Job drawing, mm, ordinate dimensions from the low corner. One solid piece. A direction names the side the tool comes from. Give positions to 0.01 mm unless a question says otherwise; leave off trailing zeros. Order: outer loops, then holes, each group sorted by start corner. A loop starts at its lowest first (then second) coordinate and runs counter-clockwise, first axis right, second up. Notation, with made-up numbers: M 45,2.25 L 59,2.25 A23 ccw 59,23.25 Z; hole C 87,-36 d11. An arc over 180 degrees is marked long. Put each result on its own line as item: value. Start each with the question number.
1) Pin check, flat tip, straight feed: pin 1 (10 mm diameter, centred on y = 46.5, z = 13.5, fed in from -X). Stop position of the tip, or through.
2) Cut at C-C (x = 10.75). Write the cut outline in (y, z).
3) Two-plate mould, pull along Z, no slides. Class the marked faces 1, 2 and 3: released by +Z, released by -Z, zero draft, split by the parting line, or undercut.
4) Tool access for the marked faces 4 and 5: list every direction of +Z, -Z, +X, -X, +Y, -Y with a clear straight run to the whole face (end or side of a thin tool).
5) Drill centre lines: line 1 (Z direction, x = 12.5, y = 47.5); line 2 (Y direction, x = 11.75, z = 49.5); line 3 (Y direction, x = 7.25, z = 46). Where is each one in solid material? Low to high. Write a range as [from, to].
6) Cut at B-B (y = 21). Write the cut outline in (x, z).
7) Cut at A-A (z = 24). Write the cut outline in (x, y), and give its area (3 significant figures).
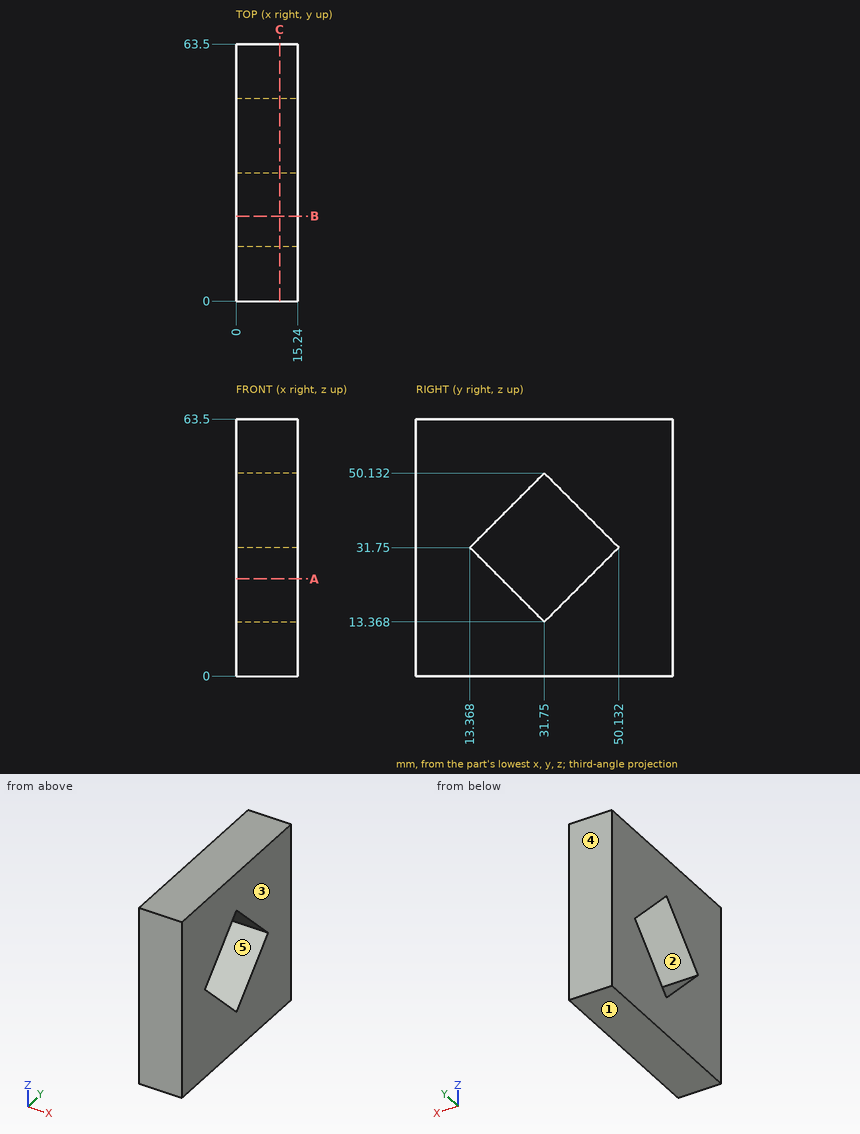
Solution:
1. pin 1: x = 0
2. outline: M 0,0 L 63.5,0 L 63.5,63.5 L 0,63.5 Z; hole M 13.37,31.75 L 31.75,13.37 L 50.13,31.75 L 31.75,50.13 Z
3. face 1: released by -Z
3. face 2: undercut
3. face 3: zero draft
4. face 4: +Z, -Z, +X, -X, +Y
4. face 5: +X, -X
5. line 1: [0, 29.12], [34.38, 63.5]
5. line 2: [0, 31.12], [32.38, 63.5]
5. line 3: [0, 27.62], [35.88, 63.5]
6. outline: M 0,0 L 15.24,0 L 15.24,24.12 L 0,24.12 Z; M 0,39.38 L 15.24,39.38 L 15.24,63.5 L 0,63.5 Z
7. outline: M 0,0 L 15.24,0 L 15.24,21.12 L 0,21.12 Z; M 0,42.38 L 15.24,42.38 L 15.24,63.5 L 0,63.5 Z
7. area: 644 mm²
